For this review, take the finished solid that the model builds, in its own axes (mm). A direction names the side the tool comes from. Round coordinates to 2 decimals unless told otherwise and drop trailing zeros. Order: outer loops, then holes, each group sorted by start corner. A loop starts at its lowest first (then second) coordinate and runs counter-clockwise, first axis right, second up. Notation, with made-up numbers: M 68.5,20 L 103.5,20 A20 cw 103.5,57 Z; hole C 21.5,77.25 d9. An arc over 180 degrees is marked long. Use a Markdown table: item, result.
from build123d import *

# Parameters (mm, degrees)
F1_DEPTH = 1828.8
F3_D     = 15.875


with BuildPart() as f1:
    # F0 (on Front) → F1 (new body)
    with BuildSketch(Plane.XZ):
        with BuildLine():
            Line((0, 100.076), (0, 0))
            Line((0, 0), (74.676, 0))
            ThreePointArc((74.676, 0), (75.753631, 0.446369), (76.2, 1.524))
            Line((76.2, 1.524), (76.2, 4.826))
            ThreePointArc((76.2, 4.826), (75.753631, 5.903631), (74.676, 6.35))
            Line((74.676, 6.35), (7.874, 6.35))
            ThreePointArc((7.874, 6.35), (6.796369, 6.796369), (6.35, 7.874))
            Line((6.35, 7.874), (6.35, 100.076))
            ThreePointArc((6.35, 100.076), (5.903631, 101.153631), (4.826, 101.6))
            Line((4.826, 101.6), (1.524, 101.6))
            ThreePointArc((1.524, 101.6), (0.446369, 101.153631), (0, 100.076))
        make_face()
    extrude(amount=F1_DEPTH)

    # F3 (through all)
    with Locations(Plane.XY.offset(6.35)):
        with Locations((41.148, -1752.6), (41.148, -1193.8), (41.148, -635), (41.148, -76.199894)):
            Hole(F3_D / 2)


solid = f1.part
Q1. Wall thickness on line 1 along X through (y, z) = (-1193.8, 3.5); line 2 along X through (y, z) = (-1365, 45): over which ranges is each line inside the solid? List them lowest first. Write a range as [from, to].
Determined:
| item | result |
|---|---|
| line 1 | x = [0, 33.21], [49.09, 76.2] |
| line 2 | x = [0, 6.35] |
Q2. Clearance check with flat-ended pins moving along their axes: pin 1 (5 mm diameter, centred on y = -1022.5, z = 62.5, fed in from +X); pin 2 (6 mm diameter, centred on x = 52.5, y = -287, fed in from +Z); pin 3 (12.5 mm diameter, centred on x = 41.15, y = -76.2, fed in from -Z). State where each tip first meets the part, or that it passes through.
Determined:
| item | result |
|---|---|
| pin 1 | stops at x = 6.35 |
| pin 2 | stops at z = 6.35 |
| pin 3 | passes through |
Q3. Machinability: for faces 1 (the flat face through (37, -902, 0)), 2 (the flat face through (6.35, -902, 53)), which of the approach directions +Z, -Z, +X, -X, +Y, -Y give a long, thin tool a straight path to every point of the face, cutting with its end or side? Answer none if there is none.
Determined:
| item | result |
|---|---|
| face 1 | -Z, +X, -X, +Y, -Y |
| face 2 | +Z, +X, +Y, -Y |
Q4. Add section A-A (z = 28). Write out the cut boundary in (x, y).
Determined:
| item | result |
|---|---|
| outline | M 0,-1828.8 L 6.35,-1828.8 L 6.35,0 L 0,0 Z |
